CAD build for the part. Positions are in the model's coordinates, mm. A direction names the side the tool comes from. Give positions to 0.01 mm unless a question says otherwise; leave off trailing zeros. Write each loop counter-clockwise with the first axis right and the second up, starting at its lowest first coordinate (ties: lowest second). Pieces come first, ordered by that corner, then holes. Notation, with made-up numbers: (35, 29) - (72, 29) arc R17 ccw to (72, 42) - close; hole circle Ø5 at (51.25, -31.75). An arc over 180 degrees is marked (long way). Put each result on its own line as item: value. Start each with the question number.
1. Tool access for faces 1 (the cylindrical face through (-2.539, 16.197, -19.334)), 2 (the flat face through (0, -23, -9)), 3 (the flat face through (2.5, -26, -9)): list every direction of +Z, -Z, +X, -X, +Y, -Y with a clear straight run to the whole face (end or side of a thin tool).
2. Wall check: line 1 (Y direction, x = 0, z = -5.75) (3 decimals); line 2 (Z direction, x = 0, y = 5.75); line 3 (Y direction, x = 0, z = -9.25) (3 decimals). Give the ranges that are in metal, low to high.
3. Cut at C-C on x = -25. List the corners of the cut face in (y, z).
4. Drop flat-ended pins along their axis: pin 1 (1.5 mm diameter, centred on y = 1, z = -21, fed in from -X); pin 2 (5 mm diameter, centred on x = -7.5, y = -10.5, fed in from -Z); pin 3 (4 mm diameter, centred on y = 1.5, z = 10, fed in from -X); pin 4 (6 mm diameter, centred on y = -5, z = 7, fed in from -X). Give the stop position or say it passes through.
5. Mould opens along Y. For faces 4 (the flat face through (0, 0, -20)), 5 (the flat face through (0, -54, -13)), 6 (the flat face through (0, -63, -3)) say: +Y half, -Y half, draft (parallel to the pull), parting line (faces both ways), or undercut.
6. Cut at B-B on z = 24. List the corners of the cut face in (x, y), and give its area (3 significant figures).
7. Cut at A-A on y = 4. List the corners of the cut face in (x, z), and give its area (3 significant figures).
from build123d import *

# Parameters (mm, degrees)
SKETCH_1_R               = 19.5
SKETCH_1_R_2             = 18
EXTRUDE_1_DEPTH          = 20
SKETCH_3_R               = 30
EXTRUDE_2_DEPTH          = 3
SKETCH_10_R              = 6
SKETCH_10_R_2            = 5
EXTRUDE_6_DEPTH          = 10
SKETCH_11_R              = 5.007506695
CUT_EXTRUDE_4_DEPTH      = 19
CUT_EXTRUDE_4_DEPTH_BACK = 10
SKETCH_15_W              = 20
SKETCH_15_H              = 60
SKETCH_15_W_2            = 13
SKETCH_15_H_2            = 25
EXTRUDE_7_DEPTH          = 1
EXTRUDE_7_DEPTH_BACK     = 2
SKETCH_16_W              = 5
SKETCH_16_H              = 5
EXTRUDE_8_DEPTH          = 10
SKETCH_18_R              = 0.875
CUT_EXTRUDE_5_DEPTH      = 10
CUT_EXTRUDE_5_DEPTH_BACK = 39
SKETCH_12_W              = 21.5
SKETCH_12_H              = 13
CUT_EXTRUDE_6_DEPTH      = 21.5
SKETCH_19_W              = 22.5
SKETCH_19_H              = 14
SKETCH_19_W_2            = 21.5
SKETCH_19_H_2            = 13
EXTRUDE_9_DEPTH          = 10
FILLET_2_R               = 1
FILLET_3_R               = 1
FILLET_4_R               = 1
FILLET_5_R               = 1
SKETCH_25_R              = 21.75
SKETCH_25_R_2            = 19.5
EXTRUDE_12_DEPTH         = 2
SKETCH_26_R              = 21.75
SKETCH_26_R_2            = 19.5
EXTRUDE_13_DEPTH         = 2


with BuildPart() as part:
    # 草圖1 → 填料-伸長1 (new body)
    with BuildSketch(Plane(origin=(0, 0, 0), x_dir=(1, 0, 0), z_dir=(0, 1, 0))):
        Circle(SKETCH_1_R)
        Circle(SKETCH_1_R_2, mode=Mode.SUBTRACT)
    extrude(amount=EXTRUDE_1_DEPTH)

    # 草圖3 → 填料-伸長2 (add)
    with BuildSketch(Plane.XZ):
        Circle(SKETCH_3_R)
    extrude(amount=EXTRUDE_2_DEPTH)

    # 草圖10 → 填料-伸長6 (add)
    with BuildSketch(Plane(origin=(0, -3, 0), x_dir=(-1, 0, 0), z_dir=(0, -1, 0))):
        with Locations((0, 11.196036894)):
            Circle(SKETCH_10_R)
        with Locations((0, 11.196036894)):
            Circle(SKETCH_10_R_2, mode=Mode.SUBTRACT)
    extrude(amount=-EXTRUDE_6_DEPTH)

    # 草圖11 → 除料-伸長4 (cut, two sides)
    with BuildSketch(Plane(origin=(0, -3, 0), x_dir=(-1, 0, 0), z_dir=(0, -1, 0))) as cut_extrude_4_sk:
        with Locations((0, 11.196036894)):
            Circle(SKETCH_11_R)
    extrude(amount=CUT_EXTRUDE_4_DEPTH, mode=Mode.SUBTRACT)
    extrude(cut_extrude_4_sk.sketch, amount=-CUT_EXTRUDE_4_DEPTH_BACK, mode=Mode.SUBTRACT)

    # 草圖15 → 填料-伸長7 (add, two sides)
    with BuildSketch(Plane.XY.offset(-3)) as extrude_7_sk:
        with Locations((0, -33)):
            Rectangle(SKETCH_15_W, SKETCH_15_H)
        with Locations((0, -40.5)):
            Rectangle(SKETCH_15_W_2, SKETCH_15_H_2, mode=Mode.SUBTRACT)
    extrude(amount=EXTRUDE_7_DEPTH)
    extrude(extrude_7_sk.sketch, amount=-EXTRUDE_7_DEPTH_BACK)

    # 草圖16 → 填料-伸長8 (add)
    with BuildSketch(Plane.XY.offset(-3)):
        with Locations((0, -25.5)):
            Rectangle(SKETCH_16_W, SKETCH_16_H)
        with Locations((0, -55.5)):
            Rectangle(SKETCH_16_W, SKETCH_16_H)
    extrude(amount=-EXTRUDE_8_DEPTH)

    # 草圖18 → 除料-伸長5 (cut, two sides)
    with BuildSketch(Plane.XY) as cut_extrude_5_sk:
        with Locations((0, -55.5)):
            Circle(SKETCH_18_R)
        with Locations((0, -25.5)):
            Circle(SKETCH_18_R)
    extrude(amount=CUT_EXTRUDE_5_DEPTH, mode=Mode.SUBTRACT)
    extrude(cut_extrude_5_sk.sketch, amount=-CUT_EXTRUDE_5_DEPTH_BACK, mode=Mode.SUBTRACT)

    # 草圖12 → 除料-伸長6 (cut)
    with BuildSketch(Plane.XZ.offset(3)):
        with Locations((0, 6.907998134)):
            Rectangle(SKETCH_12_W, SKETCH_12_H)
    extrude(amount=-CUT_EXTRUDE_6_DEPTH, mode=Mode.SUBTRACT)

    # 草圖19 → 填料-伸長9 (add)
    with BuildSketch(Plane(origin=(0, 0, 0), x_dir=(1, 0, 0), z_dir=(0, 1, 0))):
        with Locations((0, -6.907998134)):
            Rectangle(SKETCH_19_W, SKETCH_19_H)
        with Locations((0, -6.907998134)):
            Rectangle(SKETCH_19_W_2, SKETCH_19_H_2, mode=Mode.SUBTRACT)
    extrude(amount=EXTRUDE_9_DEPTH)

    # 圓角2
    fillet_2_edges = [part.edges().sort_by_distance(p)[0] for p in [
        (-11.25, 5, -0.092001866),
    ]]
    fillet(fillet_2_edges, radius=FILLET_2_R)

    # 圓角3
    fillet_3_edges = [part.edges().sort_by_distance(p)[0] for p in [
        (11.25, 5, -0.092001866),
    ]]
    fillet(fillet_3_edges, radius=FILLET_3_R)

    # 圓角4
    fillet_4_edges = [part.edges().sort_by_distance(p)[0] for p in [
        (11.25, 5, 13.907998134),
    ]]
    fillet(fillet_4_edges, radius=FILLET_4_R)

    # 圓角5
    fillet_5_edges = [part.edges().sort_by_distance(p)[0] for p in [
        (-11.25, 5, 13.907998134),
    ]]
    fillet(fillet_5_edges, radius=FILLET_5_R)

    # 草圖25 → 填料-伸長12 (add)
    with BuildSketch(Plane(origin=(0, 7, 0), x_dir=(-1, 0, 0), z_dir=(0, -1, 0))):
        Circle(SKETCH_25_R)
        Circle(SKETCH_25_R_2, mode=Mode.SUBTRACT)
    extrude(amount=EXTRUDE_12_DEPTH)

    # 草圖26 → 填料-伸長13 (add)
    with BuildSketch(Plane(origin=(0, 10.5, 0), x_dir=(-1, 0, 0), z_dir=(0, -1, 0))):
        Circle(SKETCH_26_R)
        Circle(SKETCH_26_R_2, mode=Mode.SUBTRACT)
    extrude(amount=-EXTRUDE_13_DEPTH)


solid = part.part
Report:
1. face 1: +Y
1. face 2: -Z, +X, -X
1. face 3: -Z, +X, -Y
2. line 1: y = -58 to -56.375, -54.625 to -53, -28 to -26.375, -24.625 to -23, -3 to 7
2. line 2: z = -21.75 to -18, -17.2 to -16.2, -6.19 to -5.2, -0.09 to 0.41, 13.41 to 13.91, 18 to 21.75
2. line 3: y = -58 to -56.375, -54.625 to -53, -28 to -26.375, -24.625 to -23
3. outline: (-3, -16.58) - (0, -16.58) - (0, 16.58) - (-3, 16.58) - close
4. pin 1: passes through
4. pin 2: stops at z = -5
4. pin 3: stops at x = -28.72
4. pin 4: stops at x = -29.62
5. face 4: undercut
5. face 5: draft
5. face 6: -Y half
6. outline: (-18, -3) - (18, -3) - (18, 0) - (-18, 0) - close
6. area: 108 mm²
7. outline: circle Ø39 at (0, 0); (-11.25, 0.91) arc R1 ccw to (-10.25, -0.09) - (10.25, -0.09) arc R1 ccw to (11.25, 0.91) - (11.25, 12.91) arc R1 ccw to (10.25, 13.91) - (-10.25, 13.91) arc R1 ccw to (-11.25, 12.91) - close; circle Ø12 at (0, -11.2); hole circle Ø36 at (0, 0); hole (-10.75, 0.41) - (10.75, 0.41) - (10.75, 13.41) - (-10.75, 13.41) - close; hole circle Ø10.02 at (0, -11.2)
7. area: 246 mm²
